Part print with two shaded views. Sizes in mm from the minimum x, y, z corner. Round coordinates to 2 decimals unless told otherwise and drop trailing zeros. Loops run counter-clockwise (first coordinate to the right, second up) from the corner with the lowest first, then second, coordinate; pieces in that order, holes last. Notation, with made-up numbers: M -5.75,-38 L 48.25,-38 A17 cw 48.25,-5 Z; hole C 7.5,9 d8. An arc over 180 degrees is marked long. Use a Markdown table: item, result. Add a question column.
Item 1: Pin check, flat tips, straight feed: P1, Ø2, axis at x = 48.5, z = 2, coming from the +Y side; P2, Ø0.9, axis at x = 6, y = 41.5, coming from the +Z side. Stop position of each tip, or through.
Item 2: Wall check: L1, parallel to X at y = 69.5, z = 4.05; L2, parallel to Y at x = 49.5, z = 1.85; L3, parallel to X at y = 13, z = 4.5. Give the ranges that are in metal, low to high. Write a range as from..to.
Item 3: Saw through at A-A on y = 19.5. Write the cut outline in (x, z).
Item 4: Saw through at B-B on x = 49.5. Give the number of separate pieces and of enclosed holes in the cut face, then the cut area to 3 significant figures.
Item 5: Saw through at D-D on y = 46.5. Write the cut outline in (x, z), then the cut area to 3 significant figures.
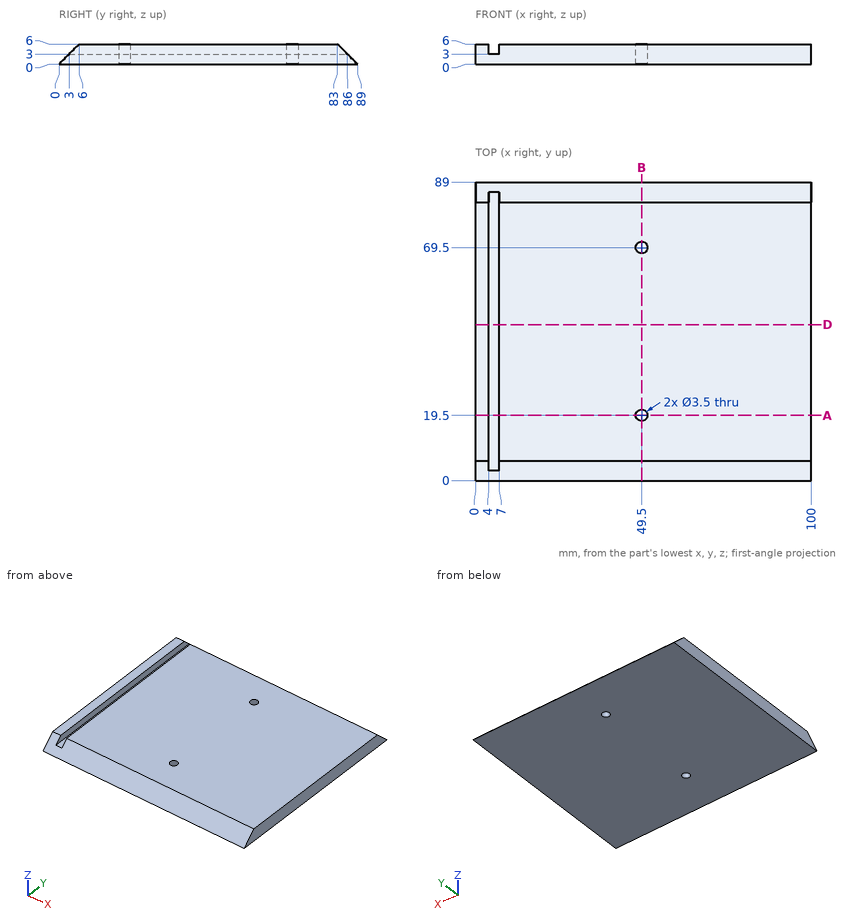
Entries:
| question | item | result |
|---|---|---|
| 1 | P1 | y = 88 |
| 1 | P2 | z = 3 |
| 2 | L1 | 0..4, 7..47.75, 51.25..100 |
| 2 | L2 | 1.85..17.75, 21.25..67.75, 71.25..87.15 |
| 2 | L3 | 0..4, 7..100 |
| 3 | outline | M 0,0 L 47.75,0 L 47.75,6 L 7,6 L 7,3 L 4,3 L 4,6 L 0,6 Z; M 51.25,0 L 100,0 L 100,6 L 51.25,6 Z |
| 4 | separate pieces | 3 |
| 4 | enclosed holes | 0 |
| 4 | area | 456 mm2 |
| 5 | outline | M 0,0 L 100,0 L 100,6 L 7,6 L 7,3 L 4,3 L 4,6 L 0,6 Z |
| 5 | area | 591 mm2 |
